Autodesk Inventor part; units mm, degrees
ref_plane "YZ Plane" through (0, 0, 0) normal (1, 0, 0) x (0, 1, 0)
ref_plane "XZ Plane" through (0, 0, 0) normal (0, 1, 0) x (-1, 0, 0)
ref_plane "XY Plane" through (0, 0, 0) normal (0, 0, 1) x (1, 0, 0)
sketch "Sketch1" plane through (0, 0, 0) normal (0, 1, 0) x (-1, 0, 0)
  line L0 (10, -10) -> (-10, -10)
  line L1 (-10, -10) -> (-10, 10)
  line L2 (-10, 10) -> (10, 10)
  line L3 (10, 10) -> (10, -10)
  line L4 (10, -10) -> (-10, 10) construction
  line L5 (-10, -10) -> (10, 10) construction
  line L6 (-15, 15) -> (15, 15)
  line L7 (15, 15) -> (15, -15)
  line L8 (15, -15) -> (-15, -15)
  line L9 (-15, -15) -> (-15, 15)
  line L10 (-15, 15) -> (15, -15) construction
  line L11 (15, 15) -> (-15, -15) construction
  circle A0 centre (12.4, 0) radius 1.5
  circle A1 centre (0, 12.5) radius 1.5
  circle A2 centre (0, -12.5) radius 1.5
  circle A3 centre (12.5, -12.5) radius 1.5
  circle A4 centre (12.5, 12.5) radius 1.5
  line L12 (0, -15) -> (0, 15)
  circle A5 centre (-12.4, 0) radius 1.5
  circle A6 centre (-12.5, -12.5) radius 1.5
  circle A7 centre (-12.5, 12.5) radius 1.5
  point P0 (0, 0)
  point P1 (10, 0)
  dimension "d0" = 20
  dimension "d1" = 20
  dimension "d4" = 30
  dimension "d5" = 30
  dimension "d6" = 3
  dimension "d7" = 3
  dimension "d8" = 3
  dimension "d9" = 12.5
  dimension "d10" = 12.4
  dimension "d11" = 12.5
  dimension "d12" = 3
  dimension "d13" = 3
  dimension "d14" = 12.5
extrude "Extrusion1" add sketch "Sketch1" along normal mid plane 10 contours L3 L2 L12 A1 L6 L7 L8 A2 L0 | L12 A2 L8 L9 L6 A1 L2 L1 L0
sketch "Sketch2" plane through (-15, 5, 15) normal (0, 0, 1) x (1, 0, 0)
  line L0 (30, 0) -> (30, -10)
  line L1 (0, 0) -> (30, 0)
  line L2 (0, -10) -> (0, 0)
  line L3 (30, -10) -> (0, -10)
  point P0 (15, -5)
  point P1 (10, -6)
  point P2 (20, -6)
  dimension "d17" = 10
  dimension "d18" = 10
hole "Hole1" at (5, -1, 15) at (-5, -1, 15) direction (0, 0, -1) diameter 2.45 depth 30
sketch "Sketch3" plane through (15, -5, -15) normal (1, 0, 0) x (0, 0, -1)
  line L0 (0, 0) -> (0, 10)
  point P0 (-15, 5)
  point P1 (-20, 5)
  point P2 (-10, 5)
  point P3 (0, 5)
  dimension "d26" = 10
  dimension "d27" = 10
hole "Hole2" at (15, 0, -5) at (15, 0, 5) direction (-1, 0, 0) diameter 2.45 depth 30
properties part number "sleeve"
Can you work these out from the model? Positions are in its coordinate system, mm. A direction names the side the tool comes from. Round coordinates to 2 decimals unless told otherwise and drop trailing zeros. Loops run counter-clockwise (first coordinate to the right, second up) from the corner with the lowest first, then second, coordinate; pieces in that order, holes last.
Item 1: Please list where these lines run through material, in increasing order: L1, parallel to Z at x = 12.5, y = -2; L2, parallel to X at y = 2.5, z = -2.25.
Item 2: Suppose I cut it at B-B, the plane z = 0. Write out the boundary of the cut face in (x, y).
Item 3: Will this pin go through, and if not, where does the flat tip stop? pin 1 Ø4 at (x, z) = (0, 12.5) entering from -Y.
Item 4: Suppose I cut it at D-D, the plane y = -2.75. State how many separate pieces and enclosed holes the cut face has, then the cut area to 3 significant figures.
Item 5: If we mould it in two halves opening along Y, with no side actions, what happens to faces 1 (the flat face through (0.2, -5, 10.2)), 2 (the cylindrical face through (12.46, 0.75, -4.03)), 3 (the flat face through (0, 0, -10))? For each: +Y half, -Y half, draft (parallel to the pull), parting line (faces both ways), or undercut.
Item 6: Which directions (+Z, -Z, +X, -X, +Y, -Y) give clear straight access to the entire face, cutting with the end or side of a thin tool? Please do faces 4 (the flat face through (0, 0, 10)), 5 (the cylindrical face through (-12.54, 0.75, -4.03)).
Item 7: Suppose I cut it at C-C, the plane x = -7.25. Write out the boundary of the cut face in (y, z), then the cut area to 3 significant figures.
Item 8: Suppose I cut it at A-A, the plane z = 12.5. Write out the boundary of the cut face in (x, y) (3 decimals).
Reported:
1. L1: z = -15 to -14, -11 to -1.5, 1.5 to 11, 14 to 15
1. L2: x = -15 to -10, 10 to 15
2. outline: (-15, -5) - (-13.9, -5) - (-13.9, 5) - (-15, 5) - close; (-10.9, -5) - (-10, -5) - (-10, 5) - (-10.9, 5) - close; (10, -5) - (10.9, -5) - (10.9, 5) - (10, 5) - close; (13.9, -5) - (15, -5) - (15, 5) - (13.9, 5) - close
3. pin 1: stops at y = -5
4. separate pieces: 1
4. enclosed holes: 9
4. area: 443 mm2
5. face 1: -Y half
5. face 2: undercut
5. face 3: draft
6. face 4: +Y, -Y
6. face 5: +X, -X
7. outline: (-5, -15) - (5, -15) - (5, -10) - (-5, -10) - close; (-5, 10) - (5, 10) - (5, 15) - (-5, 15) - close
7. area: 100 mm2
8. outline: (-15, -5) - (-14, -5) - (-14, 5) - (-15, 5) - close; (-11, -5) - (-1.5, -5) - (-1.5, 5) - (-11, 5) - close; (1.5, -5) - (11, -5) - (11, 5) - (1.5, 5) - close; (14, -5) - (15, -5) - (15, 5) - (14, 5) - close; hole circle Ø2.45 at (-5, -1); hole circle Ø2.45 at (5, -1)
